For this review, use the dimensioned drawing (mm, ordinates from the lowest corner) and the shaded views. Coordinates: 2 decimals unless noted, no trailing zeros. Write each loop counter-clockwise with the first axis right and the second up, starting at its lowest first coordinate (ties: lowest second). Pieces come first, ordered by that corner, then holes. Notation, with made-up numbers: (64.5, -35.5) - (88.5, -35.5) arc R27 cw to (88.5, -9.5) - close; hole circle Ø3 at (68.25, -15.75). An arc over 180 degrees is marked (long way). Answer as a JSON object with one key per item and string values.
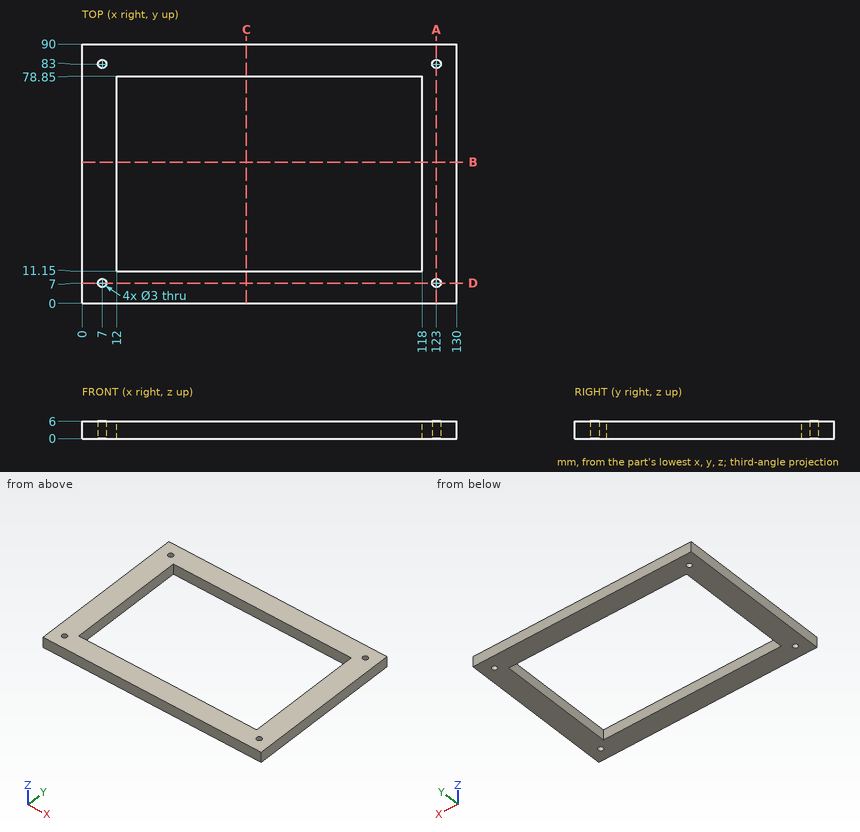
(1) Take a section at B-B, the plane y = 49. Write out the cut boundary in (x, z).
Solved:
{"outline": "(0, 0) - (12, 0) - (12, 6) - (0, 6) - close; (118, 0) - (130, 0) - (130, 6) - (118, 6) - close"}
(2) Take a section at A-A, the plane x = 123. Write out the cut boundary in (y, z), and give its area (3 significant figures).
Solved:
{"outline": "(0, 0) - (5.5, 0) - (5.5, 6) - (0, 6) - close; (8.5, 0) - (81.5, 0) - (81.5, 6) - (8.5, 6) - close; (84.5, 0) - (90, 0) - (90, 6) - (84.5, 6) - close", "area": "504 mm^2"}
(3) Take a section at C-C, the plane x = 57. Write out the cut boundary in (y, z).
Solved:
{"outline": "(0, 0) - (11.15, 0) - (11.15, 6) - (0, 6) - close; (78.85, 0) - (90, 0) - (90, 6) - (78.85, 6) - close"}
(4) Take a section at D-D, the plane y = 7. Write out the cut boundary in (x, z).
Solved:
{"outline": "(0, 0) - (5.5, 0) - (5.5, 6) - (0, 6) - close; (8.5, 0) - (121.5, 0) - (121.5, 6) - (8.5, 6) - close; (124.5, 0) - (130, 0) - (130, 6) - (124.5, 6) - close"}
(5) To check wall thickness, follow line 1 (Y direction, x = 123, z = 1.5); line 2 (Y direction, x = 22.5, z = 4.5); line 3 (X direction, y = 83, z = 1.7). State the ranges of each line that lie inside material, in increasing order. Write a range as from..to.
Solved:
{"line 1": "y = 0..5.5, 8.5..81.5, 84.5..90", "line 2": "y = 0..11.15, 78.85..90", "line 3": "x = 0..5.5, 8.5..121.5, 124.5..130"}
